Geometry: final body of the model. Coordinates: model frame, mm. A direction names the side the tool comes from. Coordinates: 2 decimals unless noted, no trailing zeros. Write each loop counter-clockwise with the first axis right and the second up, starting at its lowest first coordinate (ties: lowest second). Pieces come first, ordered by that corner, then holes.
from build123d import *

# Parameters (mm, degrees)
BOSS_EXTRUDE1_DEPTH = 8.4
CUT_EXTRUDE2_DEPTH  = 362.634640928
CUT_EXTRUDE4_DEPTH  = 362.634640928
FILLET1_R           = 4.2
SKETCH14_W          = 255.7
SKETCH14_H          = 8.4
BOSS_EXTRUDE2_DEPTH = 5


with BuildPart() as part:
    # Sketch1 → Boss-Extrude1 (new body)
    with BuildSketch(Plane.XY):
        Polygon((320.267992754, 167.253247716), (254.340919031, -26.328442922), (0, 0), (231.995455688, 171.998687612), align=None)
    extrude(amount=BOSS_EXTRUDE1_DEPTH)

    # Sketch4 → Cut-Extrude2 (cut, through all)
    with BuildSketch(Plane(origin=(84.32608447, 247.606712606, 0), x_dir=(0, 0, -1), z_dir=(-0.32238177860112127, -0.9466097341703061, 0))):
        Polygon((0, 212.749400009), (-4.2, 249.249400009), (0, 249.249400009), align=None)
    extrude(amount=CUT_EXTRUDE2_DEPTH, mode=Mode.SUBTRACT)

    # Sketch10 → Cut-Extrude4 (cut, through all)
    with BuildSketch(Plane(origin=(84.32608447, 247.606712606, 0), x_dir=(0, 0, -1), z_dir=(-0.32238177860112127, -0.9466097341703061, 0))):
        Polygon((-4.2, 249.249400009), (-8.4, 212.749400009), (-8.4, 249.249400009), align=None)
    extrude(amount=CUT_EXTRUDE4_DEPTH, mode=Mode.SUBTRACT)

    # Fillet1
    fillet1_edges = [part.edges().sort_by_distance(p)[0] for p in [
        (115.997727844, 85.999343806, 0),
        (115.997727844, 85.999343806, 8.4),
    ]]
    fillet(fillet1_edges, radius=FILLET1_R - 0.0001)  # a hair under: the kernel refuses the full size

    # Sketch14 → Boss-Extrude2 (add)
    with BuildSketch(Plane(origin=(0, 0, 0), x_dir=(0.9946848612849409, -0.10296614361312137, 0), z_dir=(-0.10296614361312136, -0.9946848612849408, 0))):
        with Locations((127.85, 4.2)):
            Rectangle(SKETCH14_W, SKETCH14_H)
    extrude(amount=BOSS_EXTRUDE2_DEPTH)


solid = part.part
Item 1: Section B-B, the plane y = -10. Output: boundary loops of the cut face in (x, z), plus the area to 3 significant figures.
Derived:
outline: (48.04, 0) - (221.34, 0) - (259.9, 4.2) - (221.34, 8.4) - (48.04, 8.4) - close
area: 1,620 mm2
Item 2: Material intervals for probe 1 along Z at (x, y) = (243, 7); probe 2 along Z at (x, y) = (275.5, 144.5); probe 3 along Y at (x, z) = (206.5, 7), sorted ascending.
Derived:
probe 1: z = 1.73 to 6.67
probe 2: z = 0.17 to 8.23
probe 3: y = -26.4 to 151.77
Item 3: Pin query (flat end, axial travel): pin 1 (1 mm diameter, centred on x = 287.5, z = 1, fed in from +Y); pin 2 (4 mm diameter, centred on x = 185, z = 5, fed in from +Y). Return the tip coordinate at first contact, or that it passes through.
Derived:
pin 1: stops at y = 169.04
pin 2: stops at y = 138.59
Item 4: Section C-C, the plane x = 300. Output: boundary loops of the cut face in (y, z).
Derived:
outline: (107.74, 4.2) - (168.34, 1.95) - (168.34, 6.45) - close
Item 5: Set-up query: faces 4 (the flat face through (268.92, 73.88, 2.07)), 5 (the flat face through (166, 58, 0)). Return all of +Z, -Z, +X, -X, +Y, -Y with unobstructed straight access to the full face (end or side cutting, diameter ignored); none if empty.
Derived:
face 4: -Z, +X
face 5: -Z, +X, -X, +Y, -Y
Item 6: Section A-A, the plane z = 6.5. Output: boundary loops of the cut face in (x, y), plus the area to 3 significant figures.
Derived:
outline: (-0.51, -4.97) - (253.83, -31.3) - (254.34, -26.33) - (233.94, -24.22) - (299.53, 168.37) - (233.07, 171.94) - (1.01, -0.1) - (0, 0) - close
area: 30,600 mm2
Item 7: Pull-direction query (Y, two-part tool) for faces 1 (the flat face through (265.706, 170.186, 4.141)), 2 (the flat face through (166, 58, 8.4)), 3 (the flat face through (269.4, 73.72, 6.27)); classes: released by +Y, released by -Y, zero draft, split by the parting line, or undercut.
Derived:
face 1: released by +Y
face 2: zero draft
face 3: undercut
